Autodesk Inventor part; units mm, degrees
ref_plane "YZ Plane" through (0, 0, 0) normal (1, 0, 0) x (0, 1, 0)
ref_plane "XZ Plane" through (0, 0, 0) normal (0, 1, 0) x (-1, 0, 0)
ref_plane "XY Plane" through (0, 0, 0) normal (0, 0, 1) x (1, 0, 0)
sketch "スケッチ1" plane through (0, 0, 0) normal (0, 0, 1) x (1, 0, 0)
  line L0 (-22, -24) -> (22, -24)
  line L1 (22, -24) -> (22, 24)
  line L2 (22, 24) -> (-22, 24)
  line L3 (-22, 24) -> (-22, -24)
  line L4 (-22, -24) -> (22, 24) construction
  line L5 (22, -24) -> (-22, 24) construction
  line L6 (-17, 15) -> (17, 15)
  line L7 (17, 15) -> (17, -19)
  line L8 (17, -19) -> (-17, -19)
  line L9 (-17, -19) -> (-17, 15)
  circle A0 centre (-17, 15) radius 3
  circle A1 centre (17, 15) radius 3
  circle A2 centre (17, -19) radius 3
  circle A3 centre (-17, -19) radius 3
  circle A4 centre (-17, 15) radius 8
  circle A5 centre (17, 15) radius 8
  circle A6 centre (17, -19) radius 8
  circle A7 centre (-17, -19) radius 8
  line L10 (-22, -24) -> (22, -24)
  line L11 (22, -24) -> (22, -28)
  line L12 (22, -28) -> (-22, -28)
  line L13 (-22, -28) -> (-22, -24)
  line L14 (-2.5, 15) -> (2.5, 15)
  line L15 (2.5, 15) -> (2.5, -19)
  line L16 (2.5, -19) -> (-2.5, -19)
  line L17 (-2.5, -19) -> (-2.5, 15)
  line L18 (10.5, 15) -> (10.5, -19)
  line L19 (5.5, -19) -> (5.5, 15)
  line L20 (18.5, 15) -> (18.5, -19)
  line L21 (13.5, -19) -> (13.5, 15)
  line L22 (-5.5, 15) -> (-5.5, -19)
  line L23 (-10.5, -19) -> (-10.5, 15)
  line L24 (2.5, 15) -> (2.5, -19)
  line L25 (-2.5, -19) -> (-2.5, 15)
  line L26 (10.5, 15) -> (10.5, -19)
  line L27 (5.5, -19) -> (5.5, 15)
  line L28 (-13.5, 15) -> (-13.5, -19)
  line L29 (-18.5, -19) -> (-18.5, 15)
  line L30 (-5.5, 15) -> (-5.5, -19)
  line L31 (-10.5, -19) -> (-10.5, 15)
  line L32 (2.5, 15) -> (2.5, -19)
  line L33 (-2.5, -19) -> (-2.5, 15)
  point P0 (0, 0)
  point P1 (-9, 15)
  point P2 (9, 15)
  point P3 (17, 7)
  point P4 (17, -11)
  point P5 (9, -19)
  point P6 (-9, -19)
  point P7 (-17, -11)
  point P8 (-17, 7)
  point P9 (22, -24)
  point P10 (0, 15)
  point P11 (-18.5, 7.1419)
  point P12 (-18.5, -11.1419)
  point P13 (-13.5, -11.8063)
  point P14 (-13.5, 7.8063)
  point P15 (-10.5, 15)
  point P16 (-10.5, -19)
  point P17 (-5.5, -19)
  point P18 (-5.5, 15)
  point P19 (13.5, 7.8063)
  point P20 (13.5, -11.8063)
  point P21 (18.5, -11.1419)
  point P22 (18.5, 7.1419)
  point P23 (5.5, 15)
  point P24 (5.5, -19)
  point P25 (10.5, -19)
  point P26 (10.5, 15)
  point P27 (-2.5, -19)
  point P28 (2.5, 15)
  point P29 (-10.5, -14.3363)
  point P30 (-10.5, 10.3363)
  point P31 (10.5, 10.3363)
  point P32 (10.5, -14.3363)
  dimension "d0" = 48
  dimension "d1" = 44
  dimension "d2" = 34
  dimension "d3" = 5
  dimension "d4" = 5
  dimension "d5" = 6
  dimension "d6" = 16
  dimension "d11" = 4
  dimension "d12" = 5
  dimension "d15" = 8
  dimension "d18" = 8
extrude "プレート1" add sketch "スケッチ1" along normal blind 1.5 contours L3 A7 L29 A3 L8 L0 | L0 A7 L13 | A7 L8 A6 L0 | L0 A6 L11 L12 L13 A7 | L3 A4 L29 A7 | A6 L8 A2 L20 L1 L0 | L0 L11 A6 | L8 L23 A7 | L3 A4 L6 A0 L29 | A7 L9 A3 L29 | A6 L18 L8 | L22 L6 L17 L8 | L8 L28 A7 L23 | A7 L28 A4 L23 | L3 L2 L1 A5 L6 A4 | L29 A0 L9 A4 | A7 L28 L8 A3 L9 | A6 L20 A5 L1 | L18 A6 L21 L8 | L8 L15 L6 L19 | L18 A5 L21 A6 | L23 L6 A4 | A4 L28 L6 L23 | L9 A0 L6 L28 A4 | A5 L20 A1 L6 L1 | L20 A2 L7 A6 | L21 A6 L7 A2 L8 | L18 L6 L21 A5 | A5 L6 L18 | A5 L7 A1 L20 | L21 L6 A1 L7 A5
sketch "スケッチ2" plane through (0, 0, 1.5) normal (0, 0, 1) x (1, 0, 0)
  line L0 (11.5, -21.5) -> (11.5, -14.8)
  line L1 (11.5, -21.5) -> (12, -21.5)
  line L2 (12, -21.5) -> (12, -24)
  line L3 (18, -24) -> (14, -24)
  line L4 (18, -14) -> (18, -24) construction
  line L5 (12.3, -14) -> (18, -14)
  circle A0 centre (12.3, -14.8) radius 0.8
  circle A1 centre (14, -23.2) radius 0.8
  line L6 (0, 0) -> (0, -10)
  circle A2 centre (-12.3, -14.8) radius 0.8
  circle A3 centre (-14, -23.2) radius 0.8
  arc A4 (11.5, -14.8) -> (12.3, -14) centre (12.3, -14.8) ccw
  line L7 (14, -24) -> (12, -24)
  circle A5 centre (14, -23.2) radius 0.8
  dimension "d21" = 1.6
  dimension "d22" = 1.6
  dimension "d25" = 2
extrude "切り取り1" cut sketch "スケッチ2" against normal blind 1.5
sketch "スケッチ3" plane through (0, 0, 1.5) normal (0, 0, 1) x (1, 0, 0)
  circle A0 centre (0, 19) radius 0.8
  circle A1 centre (-10, 19) radius 0.8
  circle A2 centre (10, 19) radius 0.8
  line L0 (-22, 24) -> (22, 24)
  point P0 (0, 0)
  point P1 (0, 24)
  dimension "d26" = 1.6
  dimension "d27" = 1.6
  dimension "d28" = 1.6
  dimension "d29" = 5
  dimension "d30" = 10
  dimension "d31" = 10
extrude "切り取り2" cut sketch "スケッチ3" against normal blind 1.5
sketch "スケッチ5" plane through (0, 0, 1.5) normal (0, 0, 1) x (1, 0, 0)
  line L0 (-32.0708, 30) -> (50, 30)
  line L1 (50, 30) -> (50, -40)
  line L2 (50, -40) -> (-32.0708, -40)
  line L3 (-32.0708, -40) -> (-32.0708, 30)
  point P0 (0, 0)
extrude "押し出し2" cut sketch "スケッチ5" against normal blind 1.2
sketch "スケッチ6" plane through (0, 0, 0.3) normal (0, 0, 1) x (1, 0, 0)
  circle A0 centre (-10, 19) radius 0.8
  circle A1 centre (0, 19) radius 0.8
  circle A2 centre (10, 19) radius 0.8
  circle A3 centre (-12.3, -14.8) radius 0.8
  circle A4 centre (12.3, -14.8) radius 0.8
  circle A5 centre (14, -23.2) radius 0.8
  circle A6 centre (-14, -23.2) radius 0.8
  line L0 (13.5, 7.8063) -> (13.5, -11.8063)
  arc A7 (13.5, 7.8063) -> (18.5, 7.1419) centre (17, 15) ccw
  line L1 (18.5, -11.1419) -> (18.5, 7.1419)
  arc A8 (18.5, -11.1419) -> (13.5, -11.8063) centre (17, -19) ccw
  arc A9 (-13.5, -11.8063) -> (-18.5, -11.1419) centre (-17, -19) ccw
  line L2 (-18.5, 7.1419) -> (-18.5, -11.1419)
  arc A10 (-18.5, 7.1419) -> (-13.5, 7.8063) centre (-17, 15) ccw
  line L3 (-13.5, -11.8063) -> (-13.5, 7.8063)
  arc A11 (10.5, -14.3363) -> (9, -19) centre (17, -19) ccw
  line L4 (5.5, -19) -> (9, -19)
  line L5 (5.5, 15) -> (5.5, -19)
  line L6 (9, 15) -> (5.5, 15)
  arc A12 (9, 15) -> (10.5, 10.3363) centre (17, 15) ccw
  line L7 (10.5, -14.3363) -> (10.5, 10.3363)
  circle A13 centre (-17, 15) radius 3
  circle A14 centre (-17, -19) radius 3
  line L8 (-2.5, -19) -> (2.5, -19)
  line L9 (-2.5, 15) -> (-2.5, -19)
  line L10 (2.5, 15) -> (-2.5, 15)
  line L11 (2.5, -19) -> (2.5, 15)
  circle A15 centre (17, -19) radius 3
  circle A16 centre (17, 15) radius 3
  line L12 (-9, -19) -> (-5.5, -19)
  arc A17 (-9, -19) -> (-10.5, -14.3363) centre (-17, -19) ccw
  line L13 (-10.5, 10.3363) -> (-10.5, -14.3363)
  arc A18 (-10.5, 10.3363) -> (-9, 15) centre (-17, 15) ccw
  line L14 (-5.5, 15) -> (-9, 15)
  line L15 (-5.5, -19) -> (-5.5, 15)
  line L16 (-22, 24) -> (22, 24)
  line L17 (-22, -28) -> (-22, 24)
  line L18 (22, -28) -> (-22, -28)
  line L19 (22, 24) -> (22, -28)
  point P0 (0, 0)
extrude "押し出し3" add sketch "スケッチ6" against normal up to surface (0.3 mm away) contours A0 | A1 | A2 | A3 | A4 | A5 | A6 | A7 L1 A8 L0 | A9 L2 A10 L3 | A11 L4 L5 L6 A12 L7 | L9 L10 L11 L8 | A17 L13 A18 L14 L15 L12
equation "\"d4\" = d3"
equation "\"d23\" = Thickness"
equation "\"d32\" = Thickness"
equation "\"d10\" = Thickness"
equation "\"BendRadius\" = Thickness"
equation "\"BendReliefWidth\" = Thickness"
equation "\"BendReliefDepth\" = 0.5 * Thickness"
equation "\"CornerReliefSize\" = 4 * Thickness"
equation "\"MinimumRemnant\" = 2 * Thickness"
equation "\"TransitionRadius\" = BendRadius"
equation "\"JacobiRadiusSize\" = BendRadius"
equation "\"GapSize\" = Thickness"
properties part number "board_setter_safety"
For this review, take the finished solid that the model builds, in its own axes (mm). Coordinates: 2 decimals unless noted, no trailing zeros. Write each loop counter-clockwise with the first axis right and the second up, starting at its lowest first coordinate (ties: lowest second). Pieces come first, ordered by that corner, then holes. Notation, with made-up numbers: (16, -14) -> (39, -14) arc R6 ccw to (39, -4) -> close; hole circle Ø1 at (24.5, 20.25). An arc over 180 degrees is marked (long way). Put each result on its own line as item: value.
Q1. Take a section at C-C, the plane y = -19. State the section outline as (x, z) points, then the cut area to 3 significant figures.
From the geometry:
outline: (-22, 0) -> (-20, 0) -> (-20, 0.3) -> (-22, 0.3) -> close; (-14, 0) -> (14, 0) -> (14, 0.3) -> (-14, 0.3) -> close; (20, 0) -> (22, 0) -> (22, 0.3) -> (20, 0.3) -> close
area: 9.60 mm2
Q2. Take a section at B-B, the plane x = 17. State the section outline as (y, z) points, then the cut area to 3 significant figures.
From the geometry:
outline: (-28, 0) -> (-22, 0) -> (-22, 0.3) -> (-28, 0.3) -> close; (-16, 0) -> (12, 0) -> (12, 0.3) -> (-16, 0.3) -> close; (18, 0) -> (24, 0) -> (24, 0.3) -> (18, 0.3) -> close
area: 12.0 mm2
Q3. Wall thickness on L1, parallel to Y at x = -17, z = 0.25; L2, parallel to Y at x = -16, z = 0.25; L3, parallel to X at y = -20.5, z = 0.25: over which ranges is each line inside the solid? List them lowest first.
From the geometry:
L1: y = -28 to -22, -16 to 12, 18 to 24
L2: y = -28 to -21.83, -16.17 to 12.17, 17.83 to 24
L3: x = -22 to -19.6, -14.4 to 14.4, 19.6 to 22
Q4. Take a section at A-A, the plane z = 0.1. State the section outline as (x, y) points, then the cut area to 3 significant figures.
From the geometry:
outline: (-22, -28) -> (22, -28) -> (22, 24) -> (-22, 24) -> close; hole circle Ø6 at (-17, -19); hole circle Ø6 at (-17, 15); hole circle Ø6 at (17, -19); hole circle Ø6 at (17, 15)
area: 2,170 mm2
Q5. The part is to be moulded in two halves that separate along Y. For faces 1 (the cylindrical face through (19.77, 16.15, 0.15)), 2 (the flat face through (0, -2, 0.3)), say which applies: +Y half, -Y half, draft (parallel to the pull), parting line (faces both ways), or undercut.
From the geometry:
face 1: undercut
face 2: draft
Q6. Clearance check with a flat-ended pin moving along its axis: pin 1 Ø5.5 at (x, y) = (-17, -19) entering from -Z. State where the tip first meets the part, or that it passes through.
From the geometry:
pin 1: passes through
